```python
from build123d import *

# Parameters (mm, degrees)
POCKET_DEPTH    = 4.501
POCKET001_DEPTH = 4.501
POCKET002_DEPTH = 4.501
POCKET003_DEPTH = 4.501


with BuildPart() as part:
    # Sketch → Revolution (revolve)
    with BuildSketch(Plane.XZ):
        with BuildLine():
            Line((0, 4.5), (1.468763, 4.5))
            ThreePointArc((1.967862, 4.030002), (1.811545, 4.364006), (1.468763, 4.5))
            Line((1.967862, 4.030002), (2.15, 1))
            Line((2.15, 1), (3.9, 1))
            Line((3.9, 1), (3.9, 4.5))
            Line((3.9, 4.5), (4.9, 4.5))
            Line((4.9, 4.5), (4.9, 0))
            Line((4.9, 0), (0, 0))
            Line((0, 0), (0, 4.5))
        make_face()
    revolve(axis=Axis((0, 0, 0), (0, 0, 1)))

    # Sketch002 (on Face6 of Revolution) → Pocket (cut, through all)
    with BuildSketch(Plane(origin=(0, 0, 0), x_dir=(1, 0, 0), z_dir=(0, 0, -1))):
        with BuildLine():
            Line((-2.15, 0), (-3.35, 0))
            ThreePointArc((-2.368808, 2.368808), (-3.094996, 1.281989), (-3.35, 0))
            Line((-2.368808, 2.368808), (-1.52028, 1.52028))
            ThreePointArc((-1.52028, 1.52028), (-1.986341, 0.822769), (-2.15, 0))
        make_face()
    extrude(amount=-POCKET_DEPTH, mode=Mode.SUBTRACT)

    # Sketch003 (on Face6 of Revolution) → Pocket001 (cut, through all)
    with BuildSketch(Plane(origin=(0, 0, 0), x_dir=(1, 0, 0), z_dir=(0, 0, -1))):
        with BuildLine():
            Line((0, 2.15), (0, 3.35))
            ThreePointArc((2.368808, 2.368808), (1.281989, 3.094996), (0, 3.35))
            Line((2.368808, 2.368808), (1.52028, 1.52028))
            ThreePointArc((1.52028, 1.52028), (0.822769, 1.986341), (0, 2.15))
        make_face()
    extrude(amount=-POCKET001_DEPTH, mode=Mode.SUBTRACT)

    # Sketch004 (on Face6 of Revolution) → Pocket002 (cut, through all)
    with BuildSketch(Plane(origin=(0, 0, 0), x_dir=(1, 0, 0), z_dir=(0, 0, -1))):
        with BuildLine():
            Line((2.15, 0), (3.35, 0))
            ThreePointArc((2.368808, -2.368808), (3.094996, -1.281989), (3.35, 0))
            Line((2.368808, -2.368808), (1.52028, -1.52028))
            ThreePointArc((1.52028, -1.52028), (1.986341, -0.822769), (2.15, 0))
        make_face()
    extrude(amount=-POCKET002_DEPTH, mode=Mode.SUBTRACT)

    # Sketch005 (on Face6 of Revolution) → Pocket003 (cut, through all)
    with BuildSketch(Plane(origin=(0, 0, 0), x_dir=(1, 0, 0), z_dir=(0, 0, -1))):
        with BuildLine():
            Line((0, -2.15), (0, -3.35))
            ThreePointArc((-2.368808, -2.368808), (-1.281989, -3.094996), (0, -3.35))
            Line((-2.368808, -2.368808), (-1.52028, -1.52028))
            ThreePointArc((-1.52028, -1.52028), (-0.822769, -1.986341), (0, -2.15))
        make_face()
    extrude(amount=-POCKET003_DEPTH, mode=Mode.SUBTRACT)


solid = part.part
```
Input: part model. Units: mm. Frame: model coordinates. A direction names the side the tool comes from. Give positions to 0.01 mm unless a question says otherwise; leave off trailing zeros. Order: outer loops, then holes, each group sorted by start corner. A loop starts at its lowest first (then second) coordinate and runs counter-clockwise, first axis right, second up. Notation, with made-up numbers: M -22,10 L -16,10 A21 cw -16,22 Z; hole C 2,34 d1. An arc over 180 degrees is marked long. One line per question, with ' | ' between items.
1) Section A-A on x = 3.75. Output: boundary loops of the cut face in (y, z).
Filled in:
outline: M -3.15,0 L 3.15,0 L 3.15,4.5 L 1.07,4.5 L 1.07,1 L -1.07,1 L -1.07,4.5 L -3.15,4.5 Z
2) Section D-D on y = 4.25. Output: boundary loops of the cut face in (x, z).
Filled in:
outline: M -2.44,0 L 2.44,0 L 2.44,4.5 L -2.44,4.5 Z
3) Section B-B on z = 1.4. Output: boundary loops of the cut face in (x, y), and give its area (3 significant figures).
Filled in:
outline: C 0,0 d9.8; C 0,0 d4.25; hole C 0,0 d7.8 | area: 41.8 mm2
4) Contact query for flat-ended pins moving along their axis: P1, Ø1, axis at y = 0.5, z = 2.5, coming from the -X side; P2, Ø0.8, axis at x = 2.5, z = 0.5, coming from the +Y side; P3, Ø2, axis at y = 3, z = 3.5, coming from the -X side; P4, Ø0.5, axis at x = -2.5, z = 0.5, coming from the -Y side. Output: stop coordinate, or through.
Filled in:
P1: stops at x = -4.9 | P2: stops at y = 4.43 | P3: stops at x = -4.47 | P4: stops at y = -4.35
5) Draft query along Y for faces 1 (the face through (4, -1, 4.5)), 2 (the face through (-1.062, -4.783, 2.218)), 3 (the face through (-3.088, -1.299, 0.493)). Return one class per face: pulls with the +Y half, pulls with the -Y half, needs draft (parallel to the pull), parting line crosses it, or undercut.
Filled in:
face 1: needs draft | face 2: parting line crosses it | face 3: undercut
6) Ray query, L1, parallel to Y at x = -1, z = 3.7; L2, parallel to Y at x = 1.25, z = 2.1; L3, parallel to X at y = 0.5, z = 4.15. Return the intervals inside material, ascending.
Filled in:
L1: y = -4.8 to -3.77, -1.72 to 1.72, 3.77 to 4.8 | L2: y = -4.74 to -3.69, -1.67 to 1.67, 3.69 to 4.74 | L3: x = -4.87 to -3.87, -1.88 to 1.88, 3.87 to 4.87
7) Access query for faces 4 (the face through (-2.87, 2.64, 2.77)), 5 (the face through (0, 0, 0)), 6 (the face through (-2.7, 0, 0.5)). Directions: +Z, -Z, +X, -X, +Y, -Y. A direction counts if a zero-diameter tool reaches every point of the face in a straight line with its end or side. Return the directions, or none.
Filled in:
face 4: +Z | face 5: -Z, +X, -X, +Y, -Y | face 6: +Z, -Z
8) Section C-C on x = -1.75. State how many separate pieces and enclosed holes the cut face has, and give its area (3 significant figures).
Filled in:
separate pieces: 3 | enclosed holes: 0 | area: 22.3 mm2
